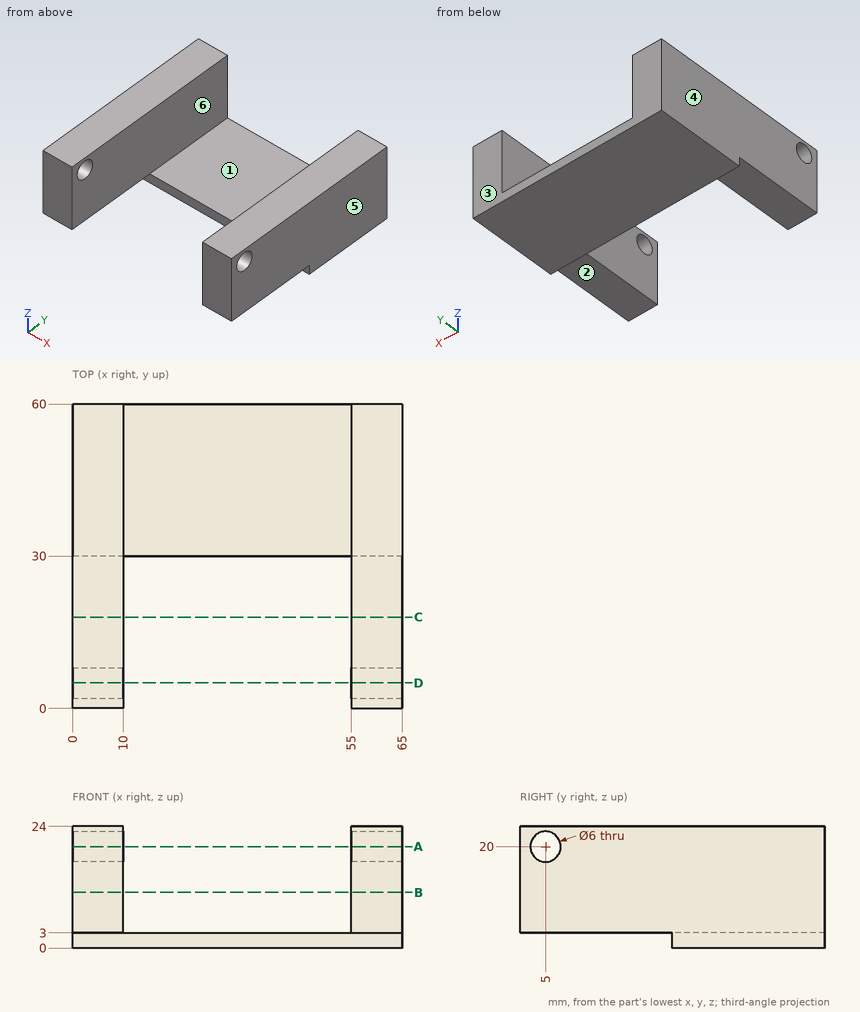
Here's the drawing with two shaded views (mm, measured from the low corner). I have some questions. A direction names the side the tool comes from. Give positions to 0.01 mm unless a question says otherwise; leave off trailing zeros. Loops run counter-clockwise (first coordinate to the right, second up) from the corner with the lowest first, then second, coordinate; pieces in that order, holes last. Notation, with made-up numbers: (85, 23.5) -> (139, 23.5) arc R20 cw to (139, 40.5) -> close; hole circle Ø8 at (-39.5, -24). An arc over 180 degrees is marked (long way). Answer as a JSON object with one key per item and string values. Group by question number.
Item 1: Thinking about a two-plate mould opening in X: for the marked faces 4, 5 and 6, which applies, pulls with the +X half, pulls with the -X half, needs draft (parallel to the pull), parting line crosses it, or undercut?
Item 2: I need wall thicknesses on L1, parallel to X at y = 43, z = 20.75; L2, parallel to Y at x = 7, z = 20; L3, parallel to Z at x = 47.5, y = 56. Which ranges of each line are inside material? Lowest first, please.
Item 3: Will these pins go through, and if not, where does the flat tip stop? pin 1 (8 mm diameter, centred on x = 11, y = 8.5, fed in from -Z); pin 2 (0.9 mm diameter, centred on x = 28, z = 1, fed in from -Y); pin 3 (15 mm diameter, centred on x = 32.5, y = 52, fed in from +Z).
Item 4: Imagine slicing it at B-B on z = 11. Write out the boundary of the cut face in (x, y).
Item 5: Imagine slicing it at D-D on y = 5. Write out the boundary of the cut face in (x, z).
Item 6: Imagine slicing it at C-C on y = 18. Write out the boundary of the cut face in (x, z), then the cut area to 3 significant figures.
Item 7: On a 3-axis mill with a long thin cutter (end or side, diameter ignored), from which of +Z, -Z, +X, -X, +Y, -Y can I reach the whole of each face in a straight line? I mean the marked faces 1, 2 and 3. Say none if no direction works.
Item 8: Imagine slicing it at A-A on z = 20. Write out the boundary of the cut face in (x, y), then the cut area to 3 significant figures.
Answer list:
{
 "1": {"face 4": "pulls with the -X half", "face 5": "pulls with the +X half", "face 6": "undercut"},
 "2": {"L1": "x = 0 to 10, 55 to 65", "L2": "y = 0 to 2, 8 to 60", "L3": "z = 0 to 3"},
 "3": {"pin 1": "stops at z = 3", "pin 2": "stops at y = 30", "pin 3": "stops at z = 3"},
 "4": {"outline": "(0, 0) -> (10, 0) -> (10, 60) -> (0, 60) -> close; (55, 0) -> (65, 0) -> (65, 60) -> (55, 60) -> close"},
 "5": {"outline": "(0, 3) -> (10, 3) -> (10, 17) -> (0, 17) -> close; (0, 23) -> (10, 23) -> (10, 24) -> (0, 24) -> close; (55, 3) -> (65, 3) -> (65, 17) -> (55, 17) -> close; (55, 23) -> (65, 23) -> (65, 24) -> (55, 24) -> close"},
 "6": {"outline": "(0, 3) -> (10, 3) -> (10, 24) -> (0, 24) -> close; (55, 3) -> (65, 3) -> (65, 24) -> (55, 24) -> close", "area": "420 mm2"},
 "7": {"face 1": "+Z, +Y, -Y", "face 2": "-Z, +X, -X, -Y", "face 3": "+Z, -Z, +X, -X, +Y"},
 "8": {"outline": "(0, 0) -> (10, 0) -> (10, 2) -> (0, 2) -> close; (0, 8) -> (10, 8) -> (10, 60) -> (0, 60) -> close; (55, 0) -> (65, 0) -> (65, 2) -> (55, 2) -> close; (55, 8) -> (65, 8) -> (65, 60) -> (55, 60) -> close", "area": "1,080 mm2"}
}
